from build123d import *

# Parameters (mm, degrees)
SKETCH1_R           = 11
BOSS_EXTRUDE1_DEPTH = 33.835
SKETCH2_R           = 6.5
BOSS_EXTRUDE2_DEPTH = 6.5
SKETCH3_R           = 5
BOSS_EXTRUDE3_DEPTH = 1
SKETCH4_R           = 3.5
BOSS_EXTRUDE4_DEPTH = 2
SKETCH5_R           = 2
BOSS_EXTRUDE5_DEPTH = 10.9


with BuildPart() as part:
    # Sketch1 → Boss-Extrude1 (new body, symmetric)
    with BuildSketch(Plane(origin=(0, 0, 0), x_dir=(1, 0, 0), z_dir=(0, 1, 0))):
        Circle(SKETCH1_R)
    extrude(amount=BOSS_EXTRUDE1_DEPTH, both=True)

    # Sketch2 → Boss-Extrude2 (add)
    with BuildSketch(Plane(origin=(0, 33.835, 0), x_dir=(1, 0, 0), z_dir=(0, 1, 0))):
        Circle(SKETCH2_R)
    extrude(amount=BOSS_EXTRUDE2_DEPTH)

    # Sketch3 → Boss-Extrude3 (add)
    with BuildSketch(Plane.XZ.offset(33.835)):
        Circle(SKETCH3_R)
    extrude(amount=BOSS_EXTRUDE3_DEPTH)

    # Sketch4 → Boss-Extrude4 (add)
    with BuildSketch(Plane(origin=(0, -34.835, 0), x_dir=(-1, 0, 0), z_dir=(0, -1, 0))):
        Circle(SKETCH4_R)
    extrude(amount=BOSS_EXTRUDE4_DEPTH)

    # Sketch5 → Boss-Extrude5 (add)
    with BuildSketch(Plane.XZ.offset(36.835)):
        Circle(SKETCH5_R)
    extrude(amount=BOSS_EXTRUDE5_DEPTH)


solid = part.part
Check sheet for the modelled part. Datum: model origin and axes. Units: mm. A direction names the side the tool comes from. Give positions to 0.01 mm unless a question says otherwise; leave off trailing zeros. Loops run counter-clockwise (first coordinate to the right, second up) from the corner with the lowest first, then second, coordinate; pieces in that order, holes last. Notation, with made-up numbers: M -38,-24.75 L -34,-24.75 A15 ccw -34,-16.75 Z; hole C 75,58.5 d1. An arc over 180 degrees is marked long. Use a Markdown table: item, result. Add a question column.
Q1. Sectioned sample at A-A, the plane x = 0. Record the cut outline in (y, z) (3 decimals), then the cut area to 3 significant figures.
Q2. Sectioned sample at B-B, the plane z = 0. Record the cut outline in (x, y) (3 decimals).
Q3. Sectioned sample at D-D, the plane x = -7.5. Record the cut outline in (y, z) (3 decimals).
Q4. Go/stop test with flat-tipped pins: pin 1 (10 mm diameter, centred on x = -8, y = 1.5, fed in from +Z); pin 2 (5 mm diameter, centred on y = -4.5, z = 6.5, fed in from -X); pin 3 (3 mm diameter, centred on y = 25.5, z = 5.5, fed in from +X). Record where each tip stops, or that it passes through.
Q5. Sectioned sample at C-C, the plane y = 2. Record the cut outline in (x, z), then the cut area to 3 significant figures.
Q6. Scan lines: line 1 along Y through (x, z) = (-7, -3.25) (3 decimals); line 2 along Y through (x, z) = (-4, 0) (3 decimals); line 3 along Z through (x, y) = (-5.75, 24.5). Record each from-to range of solid material in increasing order. Write a range as [from, to].
Q7. Tool access check on faces 1 (the flat face through (0, 40.335, 0)), 2 (the flat face through (5, 33.835, 5)), 3 (the cylindrical face through (-1.08, -34.33, -4.88)). Record the directions out of +Z, -Z, +X, -X, +Y, -Y that give a thin tool (end or side, any length) a straight path to the whole face; none if there is none.
Verdict:
| question | item | result |
|---|---|---|
| 1 | outline | M -47.735,-2 L -36.835,-2 L -36.835,-3.5 L -34.835,-3.5 L -34.835,-5 L -33.835,-5 L -33.835,-11 L 33.835,-11 L 33.835,-6.5 L 40.335,-6.5 L 40.335,6.5 L 33.835,6.5 L 33.835,11 L -33.835,11 L -33.835,5 L -34.835,5 L -34.835,3.5 L -36.835,3.5 L -36.835,2 L -47.735,2 Z |
| 1 | area | 1,640 mm^2 |
| 2 | outline | M -11,-33.835 L -5,-33.835 L -5,-34.835 L -3.5,-34.835 L -3.5,-36.835 L -2,-36.835 L -2,-47.735 L 2,-47.735 L 2,-36.835 L 3.5,-36.835 L 3.5,-34.835 L 5,-34.835 L 5,-33.835 L 11,-33.835 L 11,33.835 L 6.5,33.835 L 6.5,40.335 L -6.5,40.335 L -6.5,33.835 L -11,33.835 Z |
| 3 | outline | M -33.835,-8.047 L 33.835,-8.047 L 33.835,8.047 L -33.835,8.047 Z |
| 4 | pin 1 | z = 10.58 |
| 4 | pin 2 | x = -10.25 |
| 4 | pin 3 | x = 10.25 |
| 5 | outline | C 0,0 d22 |
| 5 | area | 380 mm^2 |
| 6 | line 1 | [-33.835, 33.835] |
| 6 | line 2 | [-34.835, 40.335] |
| 6 | line 3 | [-9.38, 9.38] |
| 7 | face 1 | +Z, -Z, +X, -X, +Y |
| 7 | face 2 | +Y |
| 7 | face 3 | -Y |
